For this review, take the finished solid that the model builds, in its own axes (mm). A direction names the side the tool comes from. Give positions to 0.01 mm unless a question says otherwise; leave off trailing zeros. Write item = value, one per line.
```python
from build123d import *

# Parameters (mm, degrees)
SKIZZE1_W                       = 80
SKIZZE1_H                       = 5.5
KOERPER_DEPTH                   = 1.8
SCHNITT_LINEAR_AUSTRAGEN1_DEPTH = 50.553348274
LINEARES_MUSTER10_COUNT         = 21
LINEARES_MUSTER10_PITCH         = 3.658
VERRUNDUNG1_R                   = 2
VERRUNDUNG2_R                   = 1


with BuildPart() as part:
    # Skizze1 → Koerper (new, symmetric)
    with BuildSketch(Plane.XY):
        with Locations((9.115418405, 2.75)):
            Rectangle(SKIZZE1_W, SKIZZE1_H)
    extrude(amount=KOERPER_DEPTH, both=True)

    # kerbe → Schnitt-Linear austragen1 (cut, symmetric)
    with BuildSketch(Plane.XY.offset(1.8)):
        Polygon((-195.870933041, 5.5), (-29.084581595, 5.5), (-28.984581595, 5.5), (-27.505581595, 3.57116725), (-27.005581595, 3.57116725), (-25.526581595, 5.5), (-25.426581595, 5.5), (141.359769852, 5.5), (141.359769852, 339.072702894), (-195.870933041, 339.072702894), align=None)
    schnitt_linear_austragen1 = extrude(amount=SCHNITT_LINEAR_AUSTRAGEN1_DEPTH, both=True, mode=Mode.SUBTRACT)

    # Lineares Muster10: Schnitt-Linear austragen1 ×21
    with Locations(*[(i * LINEARES_MUSTER10_PITCH, 0, 0) for i in range(1, LINEARES_MUSTER10_COUNT)]):
        add(schnitt_linear_austragen1, mode=Mode.SUBTRACT)

    # Verrundung1
    # the kernel refuses this fillet: 2 mm, written as the material it takes off along each edge
    with BuildSketch(Plane(origin=(-30.884581595, 5.5, -6.793746089), x_dir=(1, 0, 0), z_dir=(0, 0, 1))) as verrundung1_piece_1:
        with BuildLine():
            CenterArc((2, -1.997498436), VERRUNDUNG1_R, 92.865983983, 87.134016017)
            Line((0, -1.997498436), (-0.04, -1.997498436))
            Line((-0.04, -1.997498436), (-0.04, 0))
            Line((-0.04, 0), (0, 0.04))
            ThreePointArc((0, 0.04), (0.95, 0.04), (1.898, 0.039949969))
            Line((1.898, 0.039949969), (1.9, 0))
        make_face()
    extrude(amount=13.587492178, mode=Mode.SUBTRACT)

    # Verrundung2
    verrundung2_edges = [part.edges().sort_by_distance(p)[0] for p in [
        (49.115418405, 5.5, 0),
    ]]
    fillet(verrundung2_edges, radius=VERRUNDUNG2_R)


solid = part.part
```
(1) To check wall thickness, follow probe 1 along Y at (x, z) = (33, -1.35); probe 2 along Y at (x, z) = (2, -0.15). State the ranges of each line that lie inside material, in increasing order.
Answers below:
probe_1 = 0 to 5.5
probe_2 = 0 to 3.57
(2) The part is to be moulded in two halves that separate along X. For faces 1 (the face through (49.115, 2, 0)), 2 (the face through (44.905, 4.549, 0.025)), 3 (the face through (9, 2, -1.8)), 4 (the face through (-30.885, 2, 0)), say which applies: released by +X, released by -X, zero draft, split by the parting line, or undercut.
Answers below:
face_1 = released by +X
face_2 = undercut
face_3 = zero draft
face_4 = released by -X
(3) Tool access review of faces 5 (the face through (9, 0, 0)), 6 (the face through (26.615, 4.549, 0.025)): name each direction out of +Z, -Z, +X, -X, +Y, -Y from which nothing blocks a thin tool from reaching the whole face with its end or side.
Answers below:
face_5 = +Z, -Z, +X, -X, -Y
face_6 = +Z, -Z, +Y
(4) For pin 1 (0.6 mm diameter, centred on x = 16.5, z = 0, fed in from +Y); pin 2 (0.6 mm diameter, centred on x = 2, z = 0.5, fed in from +Y); pin 3 (0.6 mm diameter, centred on x = -2, z = 0, fed in from +Y), all flat-tipped, find the tip position at first contact; note any pin that passes through.
Answers below:
pin_1 = 3.82
pin_2 = 3.65
pin_3 = 4.09
